The listing builds one solid part. Answer for the finished solid, in the listing's coordinates (mm). A direction names the side the tool comes from. Round coordinates to 2 decimals unless told otherwise and drop trailing zeros. Write each loop counter-clockwise with the first axis right and the second up, starting at its lowest first coordinate (ties: lowest second). Pieces come first, ordered by that corner, then holes. Notation, with made-up numbers: M -38,46.5 L -23,46.5 A22 ccw -23,79.5 Z; hole C -25.5,3 d11. An arc over 180 degrees is marked long. Write each question's results on one line, items separated by ' | '.
from build123d import *

# Parameters (mm, degrees)
BOX003_W          = 30
BOX003_H          = 8.8
BOX003_DEPTH      = 16
CYLINDER001_R     = 1.5
CYLINDER001_DEPTH = 9
CYLINDER_R        = 2.55
CYLINDER_DEPTH    = 9
BOX002_W          = 32
BOX002_H          = 103.5
BOX002_DEPTH      = 2
BOX001_W          = 37.4
BOX001_H          = 125.4
BOX001_DEPTH      = 14
BOX_W             = 40
BOX_H             = 128
BOX_DEPTH         = 16


with BuildPart() as connector_cutout:
    # Box003 → Box003 (new body)
    with BuildSketch(Plane(origin=(2.5, 119.2, 0), x_dir=(1, 0, 0), z_dir=(0, 0, 1))):
        with Locations((15, 4.4)):
            Rectangle(BOX003_W, BOX003_H)
    extrude(amount=BOX003_DEPTH)


with BuildPart() as cylinder001:
    # Cylinder001 → Cylinder001 (new body)
    with BuildSketch(Plane(origin=(4.5, 3.8, 0), x_dir=(1, 0, 0), z_dir=(0, 0, 1))):
        Circle(CYLINDER001_R)
    extrude(amount=CYLINDER001_DEPTH)


with BuildPart() as clone003:
    # Clone003 base: copy of Cylinder001
    add(cylinder001.part)


with BuildPart() as clone003_1:
    # Clone003 placement: moved
    add(clone003.part.moved(Location((31, 0, 0))))


with BuildPart() as clone004:
    # Clone004 base: copy of Cylinder001
    add(cylinder001.part)


with BuildPart() as clone004_1:
    # Clone004 placement: moved
    add(clone004.part.moved(Location((0, 113, 0))))


with BuildPart() as board_drills:
    # Clone005 base: copy of Cylinder001
    add(cylinder001.part)


with BuildPart() as board_drills_1:
    # Clone005 placement: moved
    add(board_drills.part.moved(Location((31, 113, 0))))

    # Fusion001: union Clone003, Clone004, Cylinder001
    add(clone003_1.part)
    add(clone004_1.part)
    add(cylinder001.part)


with BuildPart() as cylinder:
    # Cylinder → Cylinder (new body)
    with BuildSketch(Plane(origin=(4.5, 3.8, 0), x_dir=(1, 0, 0), z_dir=(0, 0, 1))):
        Circle(CYLINDER_R)
    extrude(amount=CYLINDER_DEPTH)


with BuildPart() as clone:
    # Clone base: copy of Cylinder
    add(cylinder.part)


with BuildPart() as clone_1:
    # Clone placement: moved
    add(clone.part.moved(Location((31, 0, 0))))


with BuildPart() as clone002:
    # Clone002 base: copy of Cylinder
    add(cylinder.part)


with BuildPart() as clone002_1:
    # Clone002 placement: moved
    add(clone002.part.moved(Location((31, 113, 0))))


with BuildPart() as clone001:
    # Clone001 base: copy of Cylinder
    add(cylinder.part)


with BuildPart() as clone001_1:
    # Clone001 placement: moved
    add(clone001.part.moved(Location((0, 113, 0))))


with BuildPart() as screen_cutout:
    # Box002 → Box002 (new body)
    with BuildSketch(Plane(origin=(4, 6.3, 0), x_dir=(1, 0, 0), z_dir=(0, 0, 1))):
        with Locations((16, 51.75)):
            Rectangle(BOX002_W, BOX002_H)
    extrude(amount=BOX002_DEPTH)


with BuildPart() as cube001:
    # Box001 → Box001 (new body)
    with BuildSketch(Plane(origin=(1.3, 1.3, 2), x_dir=(1, 0, 0), z_dir=(0, 0, 1))):
        with Locations((18.7, 62.7)):
            Rectangle(BOX001_W, BOX001_H)
    extrude(amount=BOX001_DEPTH)


with BuildPart() as case_with_connector_cutout:
    # Box → Box (new body)
    with BuildSketch(Plane.XY):
        with Locations((20, 64)):
            Rectangle(BOX_W, BOX_H)
    extrude(amount=BOX_DEPTH)

    # Cut: cut Cube001
    add(cube001.part, mode=Mode.SUBTRACT)

    # Cut001: cut Screen cutout
    add(screen_cutout.part, mode=Mode.SUBTRACT)

    # Fusion: union Clone, Clone002, Clone001, Cylinder
    add(clone_1.part)
    add(clone002_1.part)
    add(clone001_1.part)
    add(cylinder.part)

    # Cut002: cut Board drills
    add(board_drills_1.part, mode=Mode.SUBTRACT)

    # Cut003: cut Connector cutout
    add(connector_cutout.part, mode=Mode.SUBTRACT)


solid = case_with_connector_cutout.part
1) Section C-C (y = 53) is taken. Determine the outline of the cut face in (x, z).
Return value:
outline: M 0,0 L 4,0 L 4,2 L 1.3,2 L 1.3,16 L 0,16 Z; M 36,0 L 40,0 L 40,16 L 38.7,16 L 38.7,2 L 36,2 Z
2) Section B-B (y = 3.8) is taken. Determine the outline of the cut face in (x, z).
Return value:
outline: M 0,0 L 3,0 L 3,9 L 1.95,9 L 1.95,2 L 1.3,2 L 1.3,16 L 0,16 Z; M 6,0 L 34,0 L 34,9 L 32.95,9 L 32.95,2 L 7.05,2 L 7.05,9 L 6,9 Z; M 37,0 L 40,0 L 40,16 L 38.7,16 L 38.7,2 L 38.05,2 L 38.05,9 L 37,9 Z
3) Section D-D (z = 7) is taken. Determine the outline of the cut face in (x, y), then the cut area to 3 significant figures.
Return value:
outline: M 0,0 L 40,0 L 40,128 L 32.5,128 L 32.5,126.7 L 38.7,126.7 L 38.7,1.3 L 36,1.3 A2.55 ccw long 35,1.3 L 5,1.3 A2.55 ccw long 4,1.3 L 1.3,1.3 L 1.3,126.7 L 2.5,126.7 L 2.5,128 L 0,128 Z; M 3.64,119.2 A2.55 ccw long 5.36,119.2 Z; C 35.5,116.8 d5.1; hole C 4.5,3.8 d3; hole C 4.5,116.8 d3; hole C 35.5,3.8 d3; hole C 35.5,116.8 d3 | area: 444 mm²
4) Section A-A (x = 14.5) is taken. Determine the outline of the cut face in (y, z).
Return value:
outline: M 0,0 L 6.3,0 L 6.3,2 L 1.3,2 L 1.3,16 L 0,16 Z; M 109.8,0 L 119.2,0 L 119.2,2 L 109.8,2 Z
5) The mould has two halves that part along Y. Classify faces 1 (the face through (36, 126.7, 9)), 2 (the face through (15, 119.2, 1)), 3 (the face through (4.4, 114.25, 5.45)), 4 (the face through (20, 0, 8)): +Y half, -Y half, draft (parallel to the pull), parting line (faces both ways), or undercut.
Return value:
face 1: undercut | face 2: +Y half | face 3: undercut | face 4: -Y half
6) A tool of negligible diameter and unlimited length cuts with its end or side. For faces 5 (the face through (1, 64, 16)), 6 (the face through (2.5, 127, 5)), 7 (the face through (1.3, 63, 9)), 8 (the face through (5.306, 5.065, 4.437)), from which of +Z, -Z, +X, -X, +Y, -Y can it reach the whole face along a straight path? Write none if from no direction.
Return value:
face 5: +Z, +X, -X, +Y, -Y | face 6: +Z, -Z, +Y | face 7: +Z | face 8: +Z, -Z
7) Each of these flat-tipped pins is pushed along its axis until it touches: pin 1 (4 mm diameter, centred on x = 5, y = 117.5, fed in from +Z); pin 2 (1.5 mm diameter, centred on x = 23, y = 4.5, fed in from +Z). Where does it stop, or does it pass through?
Return value:
pin 1: z = 9 | pin 2: z = 2
8) Find the intervals of material crossed by line 1 (Y direction, x = 4.5, z = 6); line 2 (X direction, y = 116.8, z = 7); line 3 (Y direction, x = 35.5, z = 6.5), in increasing order.
Return value:
line 1: 0 to 2.3, 5.3 to 6.35, 114.25 to 115.3, 118.3 to 119.2 | line 2: 0 to 1.3, 1.95 to 3, 6 to 7.05, 32.95 to 34, 37 to 38.05, 38.7 to 40 | line 3: 0 to 2.3, 5.3 to 6.35, 114.25 to 115.3, 118.3 to 119.35, 126.7 to 128
